Input: part model. Units: mm. Frame: model coordinates. A direction names the side the tool comes from. Coordinates: 2 decimals unless noted, no trailing zeros. Write each loop counter-clockwise with the first axis right and the second up, starting at its lowest first coordinate (ties: lowest second). Pieces come first, ordered by that corner, then holes. Notation, with made-up numbers: (56, 80.25) - (73, 80.25) arc R22 ccw to (73, 110.25) - close; hole circle Ø6 at (-14.5, 29.5). An arc over 180 degrees is marked (long way). Put each result on its own line as item: value. Start each with the question number.
1. Pin query (flat end, axial travel): pin 1 (4 mm diameter, centred on x = 35.5, z = -4.5, fed in from +Y); pin 2 (4.5 mm diameter, centred on x = 2, y = -9, fed in from -Z); pin 3 (5 mm diameter, centred on x = 19, z = 17, fed in from -Y); pin 4 (3 mm diameter, centred on y = -5.5, z = 29.5, fed in from -X). Return the tip coordinate at first contact, or that it passes through.
2. Cut plane D-D, the plane x = 27. Return loops of the section in (y, z).
3. Cut plane A-A, the plane y = -7.75. Return loops of the section in (x, z).
4. Access query for faces 1 (the flat face through (-6, -12.7, 39)), 2 (the flat face through (8.164, -7.549, 47.234)). Directions: +Z, -Z, +X, -X, +Y, -Y. A direction counts if a zero-diameter tool reaches every point of the face in a straight line with its end or side. Return the directions, or none.
5. Cut plane B-B, the plane x = -8. Return loops of the section in (y, z), and give its area (3 significant figures).
6. Pull-direction query (X, two-part tool) for faces 3 (the flat face through (27.973, -1.252, -54.676)), 4 (the cylindrical face through (6.94, -7.549, 41.344)), 5 (the flat face through (0, -12.7, 37)), 6 (the flat face through (-26.464, -1.252, -54.273)); classes: released by +X, released by -X, zero draft, split by the parting line, or undercut.
7. Line query: line 1 (X direction, y = -8.5, z = 36); line 2 (Z direction, x = 8, y = -4.5); line 3 (Z direction, x = -1, y = -10.75). Output: solid intervals per line, ascending.
8. Cut plane C-C, the plane z = -7. Return loops of the section in (x, y).
from build123d import *

# Parameters (mm, degrees)
F1_DEPTH  = 12.7
F2_DEPTH  = 2.54
F3_DEPTH  = 7.62
F4_DEPTH  = 2.54
F5_DEPTH  = 2.54
F6_DEPTH  = 2.54
F7_DEPTH  = 2.54
F8_DEPTH  = 2.54
F9_DEPTH  = 2.54
F10_R     = 16.3446931482
F10_R_2   = 13.4473820184
F10_R_3   = 3.0169302384
F10_R_4   = 3.1385421842
F10_R_5   = 3.2190410071
F11_DEPTH = 25.4
F12_DEPTH = 19.05
F13_DEPTH = 6.35
F14_DEPTH = 2.54
F15_DEPTH = 2.54
F16_DEPTH = 2.54


with BuildPart() as f1:
    # F0 (on Front) → F1 (new body)
    with BuildSketch(Plane.XZ):
        Polygon((59.2296272516, 26.558874175), (0, 68.5641244054), (-54.7846257687, 26.558874175), (-54.7846257687, -40.5606217682), (0, -72.7868750691), (59.2296272516, -40.5606217682), align=None)
    extrude(amount=F1_DEPTH)

    # F2 (cut): a face of the model
    f2_faces = [f1.faces().sort_by_distance(p)[0] for p in [
        (1.9587071028, -12.7, -4.2659517496),
    ]]
    extrude(f2_faces, amount=-F2_DEPTH, mode=Mode.SUBTRACT)

    # F3 (cut): a face of the model
    f3_faces = [f1.faces().sort_by_distance(p)[0] for p in [
        (1.9587071028, -10.16, -4.2659517496),
    ]]
    extrude(f3_faces, amount=-F3_DEPTH, mode=Mode.SUBTRACT)

    # F4 (cut): a face of the model
    f4_faces = [f1.faces().sort_by_distance(p)[0] for p in [
        (29.6148136258, -1.27, 47.5614992902),
    ]]
    extrude(f4_faces, amount=-F4_DEPTH, mode=Mode.SUBTRACT)

    # F5 (cut): a face of the model
    f5_faces = [f1.faces().sort_by_distance(p)[0] for p in [
        (-27.3923128843, -1.27, 47.5614992902),
    ]]
    extrude(f5_faces, amount=-F5_DEPTH, mode=Mode.SUBTRACT)

    # F6 (cut): a face of the model
    f6_faces = [f1.faces().sort_by_distance(p)[0] for p in [
        (59.2296272516, -1.27, -7.0008737966),
    ]]
    extrude(f6_faces, amount=-F6_DEPTH, mode=Mode.SUBTRACT)

    # F7 (cut): a face of the model
    f7_faces = [f1.faces().sort_by_distance(p)[0] for p in [
        (-54.7846257687, -1.27, -7.0008737966),
    ]]
    extrude(f7_faces, amount=-F7_DEPTH, mode=Mode.SUBTRACT)

    # F8 (cut): a face of the model
    f8_faces = [f1.faces().sort_by_distance(p)[0] for p in [
        (-27.3923128843, -1.27, -56.6737484187),
    ]]
    extrude(f8_faces, amount=-F8_DEPTH, mode=Mode.SUBTRACT)

    # F9 (cut): a face of the model
    f9_faces = [f1.faces().sort_by_distance(p)[0] for p in [
        (29.6148136258, -1.27, -56.6737484187),
    ]]
    extrude(f9_faces, amount=-F9_DEPTH, mode=Mode.SUBTRACT)

    # F10 (on face) → F11 (join)
    with BuildSketch(Plane.XZ.offset(2.54)):
        with Locations((0.4653159413, 42.5413995981)):
            Circle(F10_R)
        with Locations((0.4653159413, 42.5413995981)):
            Circle(F10_R_2, mode=Mode.SUBTRACT)
        Polygon((5.7624652982, 51.0174520314), (1.3005869696, 43.022621423), (10.498451069, 43.5544140637), align=None)
        with Locations((7.332497742, 38.3531376719)):
            Circle(F10_R_3)
        Polygon((4.8724082299, 33.4170944989), (0.3896932758, 41.4243862033), (-4.0930220857, 33.4170944989), align=None)
        with Locations((-6.2807253562, 38.5114327073)):
            Circle(F10_R_4)
        Polygon((-5.2216826007, 50.936318934), (-9.8047619686, 43.5544140637), (-0.6910812808, 43.0121421814), align=None)
        with Locations((0.4653159413, 50.0668436289)):
            Circle(F10_R_5)
    extrude(amount=F11_DEPTH)

    # F12 (cut): faces of the model
    f12_faces = [f1.faces().sort_by_distance(p)[0] for p in [
        (-15.4170794725, -27.94, 42.5413995981),
        (0.38969314, -27.94, 36.0861917337),
        (7.332497742, -27.94, 38.3531376719),
        (5.8538344456, -27.94, 45.8648291727),
        (-5.2391752834, -27.94, 45.8342917264),
        (-6.2807253562, -27.94, 38.5114327073),
        (0.4653159413, -27.94, 50.0668436289),
    ]]
    extrude(f12_faces, amount=-F12_DEPTH, mode=Mode.SUBTRACT)

    # F13 (add): faces of the model
    f13_faces = [f1.faces().sort_by_distance(p)[0] for p in [
        (-15.4170794725, -8.89, 42.5413995981),
        (7.332497742, -8.89, 38.3531376719),
        (5.8538344456, -8.89, 45.8648291727),
        (0.4653159413, -8.89, 50.0668436289),
        (-5.2391752834, -8.89, 45.8342917264),
        (-6.2807253562, -8.89, 38.5114327073),
        (0.38969314, -8.89, 36.0861917337),
    ]]
    extrude(f13_faces, amount=F13_DEPTH)

    # F14 (cut): faces of the model
    f14_faces = [f1.faces().sort_by_distance(p)[0] for p in [
        (-15.4170794725, -15.24, 42.5413995981),
        (7.332497742, -15.24, 38.3531376719),
        (5.8538344456, -15.24, 45.8648291727),
        (0.4653159413, -15.24, 50.0668436289),
        (-5.2391752834, -15.24, 45.8342917264),
        (-6.2807253562, -15.24, 38.5114327073),
        (0.38969314, -15.24, 36.0861917337),
    ]]
    extrude(f14_faces, amount=-F14_DEPTH, mode=Mode.SUBTRACT)

    # F15 (cut): faces of the model
    f15_faces = [f1.faces().sort_by_distance(p)[0] for p in [
        (5.8538344456, -12.7, 45.8648291727),
        (0.4653159413, -12.7, 50.0668436289),
        (7.332497742, -12.7, 38.3531376719),
        (0.38969314, -12.7, 36.0861917337),
        (-5.2391752834, -12.7, 45.8342917264),
        (-6.2807253562, -12.7, 38.5114327073),
        (-15.4170794725, -12.7, 42.5413995981),
    ]]
    extrude(f15_faces, amount=-F15_DEPTH, mode=Mode.SUBTRACT)

    # F16 (add): faces of the model
    f16_faces = [f1.faces().sort_by_distance(p)[0] for p in [
        (0.4653159413, -10.16, 50.0668436289),
        (5.8538344456, -10.16, 45.8648291727),
        (7.332497742, -10.16, 38.3531376719),
        (0.38969314, -10.16, 36.0861917337),
        (-5.2391752834, -10.16, 45.8342917264),
        (-6.2807253562, -10.16, 38.5114327073),
        (-15.4170794725, -10.16, 42.5413995981),
    ]]
    extrude(f16_faces, amount=F16_DEPTH)


solid = f1.part
Report:
1. pin 1: stops at y = 0
1. pin 2: stops at z = 26.2
1. pin 3: stops at y = -2.54
1. pin 4: stops at x = -11.11
2. outline: (-2.54, -55.2) - (0, -55.2) - (0, 46.3) - (-2.54, 46.3) - close
3. outline: circle Ø32.69 at (0.47, 42.54); (-9.8, 43.55) - (-0.69, 43.01) - (-5.22, 50.94) - close; circle Ø6.28 at (-6.28, 38.51); (-4.09, 33.42) - (4.87, 33.42) - (0.39, 41.42) - close; circle Ø6.44 at (0.47, 50.07); (1.3, 43.02) - (10.5, 43.55) - (5.76, 51.02) - close; circle Ø6.03 at (7.33, 38.35); hole circle Ø26.89 at (0.47, 42.54)
4. face 1: +Z, -Z, +X, -X, -Y
4. face 2: -Y
5. outline: (-12.7, 28.56) - (-2.54, 28.56) - (-2.54, -65.13) - (0, -65.13) - (0, 59.23) - (-2.54, 59.23) - (-2.54, 56.52) - (-12.7, 56.52) - (-12.7, 52.99) - (-2.54, 52.99) - (-2.54, 46.46) - (-12.7, 46.46) - (-12.7, 43.45) - (-2.54, 43.45) - (-2.54, 41.14) - (-12.7, 41.14) - (-12.7, 35.89) - (-2.54, 35.89) - (-2.54, 32.09) - (-12.7, 32.09) - close
5. area: 472 mm^2
6. face 3: released by +X
6. face 4: undercut
6. face 5: zero draft
6. face 6: released by -X
7. line 1: x = -14.51 to -11.28, -8.16 to -4.4, -2.65 to 3.43, 5.44 to 9.22, 12.21 to 15.44
7. line 2: z = 28.04 to 31.4, 35.41 to 41.3, 43.41 to 47.49, 53.68 to 57.05
7. line 3: z = 26.26 to 29.17, 33.42 to 38.94, 43.03 to 43.55, 47.2 to 52.93, 55.91 to 58.82
8. outline: (-52.24, -2.54) - (56.69, -2.54) - (56.69, 0) - (-52.24, 0) - close
